Geometry: final body of the model. Coordinates: model frame, mm. A direction names the side the tool comes from. Give positions to 0.01 mm unless a question says otherwise; leave off trailing zeros. Order: outer loops, then holes, each group sorted by start corner. A loop starts at its lowest first (then second) coordinate and runs counter-clockwise, first axis right, second up. Notation, with made-up numbers: (24, 45.25) - (75, 45.25) arc R8 ccw to (75, 55.25) - close; hole circle Ø10 at (43, 38). An arc over 180 degrees is marked (long way). Use one line per item in the form item = value.
from build123d import *

# Parameters (mm, degrees)
F0_W     = 13
F0_H     = 2
F1_DEPTH = 40
F2_R     = 0.99999


# Not quite as in the source:
# - a fillet or chamfer is up to 0.001 mm smaller than in the source, because OpenCascade refuses the exact size


with BuildPart() as f1:
    # F0 (on Top) → F1 (new body)
    with BuildSketch(Plane.XY):
        Polygon((-24.5838956386, 17.7643506003), (-26.5838956386, 17.7643506003), (-26.5838956386, -12.2356493997), (-24.5838956386, -12.2356493997), (-24.5838956386, -10.2356493997), align=None)
        with Locations((-18.0838956386, -11.2356493997)):
            Rectangle(F0_W, F0_H)
        Polygon((-11.5838956386, 37.7643506003), (-11.5838956386, -10.2356493997), (-11.5838956386, -12.2356493997), (-9.5838956386, -12.2356493997), (-9.5838956386, 37.7643506003), align=None)
    extrude(amount=F1_DEPTH)

    # F2 (radius 1 in the source; OpenCascade refuses exactly that, so slightly less here)
    f2_edges = [f1.edges().sort_by_distance(p)[0] for p in [
        (-26.583896, 17.764351, 20),
        (-24.583896, 17.764351, 20),
        (-11.583896, 37.764351, 20),
        (-26.583896, -12.235649, 20),
        (-24.583896, -10.235649, 20),
        (-11.583896, -10.235649, 20),
    ]]
    fillet(f2_edges, radius=F2_R)


solid = f1.part
(1) Pull-direction query (X, two-part tool) for faces 1 (the face through (-10, 37.764, 20)), 2 (the face through (-18, -10.236, 20)), 3 (the face through (-26.299, -11.935, 20.28)); classes: released by +X, released by -X, zero draft, split by the parting line, or undercut.
Computed values:
face_1 = zero draft
face_2 = undercut
face_3 = released by -X
(2) Cut plane C-C on x = -16.75. Output: boundary loops of the cut face in (y, z), plus the area to 3 significant figures.
Computed values:
outline = (-12.24, 0) - (-10.24, 0) - (-10.24, 40) - (-12.24, 40) - close
area = 80.0 mm²
(3) Ray query, line 1 along X through (y, z) = (6, 5.5); line 2 along X through (y, z) = (20, 34.5); line 3 along Y through (x, z) = (-22.5, 14.5). Return the intervals inside material, ascending.
Computed values:
line_1 = -26.58 to -24.58, -11.58 to -9.58
line_2 = -11.58 to -9.58
line_3 = -12.24 to -10.24
(4) Contact query for flat-ended pins moving along their axis: pin 1 Ø10 at (x, y) = (-20.5, 28.5) entering from -Z; pin 2 Ø5 at (y, z) = (27.5, 23.5) entering from -X; pin 3 Ø12 at (y, z) = (23, 11.5) entering from -X; pin 4 Ø5 at (x, z) = (-23.5, 24.5) entering from +Y. Output: stop coordinate, or through.
Computed values:
pin_1 = through
pin_2 = -11.58
pin_3 = -26.56
pin_4 = 17.76
(5) Cut plane A-A on y = 12.5. Output: boundary loops of the cut face in (x, z).
Computed values:
outline = (-26.58, 0) - (-24.58, 0) - (-24.58, 40) - (-26.58, 40) - close; (-11.58, 0) - (-9.58, 0) - (-9.58, 40) - (-11.58, 40) - close
(6) Cut plane D-D on y = 34. Output: boundary loops of the cut face in (x, z), plus the area to 3 significant figures.
Computed values:
outline = (-11.58, 0) - (-9.58, 0) - (-9.58, 40) - (-11.58, 40) - close
area = 80.0 mm²
(7) Reachability of faces 4 (the face through (-26.584, 3, 20)), 5 (the face through (-24.584, 4, 20)) from +Z, -Z, +X, -X, +Y, -Y: full face, straight path, thin tool, end or side. Return the list, or none.
Computed values:
face_4 = +Z, -Z, -X, +Y, -Y
face_5 = +Z, -Z, +Y
